Can you work these out from the model? Positions are in its coordinate system, mm. Give positions to 0.01 mm unless a question says otherwise; leave off trailing zeros. Write each loop counter-clockwise with the first axis right and the second up, starting at its lowest first coordinate (ties: lowest second). Pieces come first, ordered by that corner, then holes. Notation, with made-up numbers: (-34.75, 12.25) -> (-11.75, 12.25) arc R27 ccw to (-11.75, 33.25) -> close; hole circle Ø2 at (75, 10.5). An arc over 180 degrees is marked (long way). One line per item, written item: value.
from build123d import *

# Parameters (mm, degrees)
SKETCH3_R           = 19.3675
BOSS_EXTRUDE2_DEPTH = 50.8


with BuildPart() as part:
    # Sketch3 → Boss-Extrude2 (new body)
    with BuildSketch(Plane(origin=(0, 0, 0), x_dir=(1, 0, 0), z_dir=(0, 1, 0))):
        Circle(SKETCH3_R)
        with BuildLine():
            Line((1.905, 12.877355367), (1.905, 10.63625))
            Line((1.905, 10.63625), (-1.905, 10.63625))
            Line((-1.905, 10.63625), (-1.905, 12.877355367))
            ThreePointArc((-1.905, 12.877355367), (-4.981581581, 12.026601814), (-7.758626886, 10.452703722))
            Line((-7.758626886, 10.452703722), (-6.173926083, 8.86800292))
            Line((-6.173926083, 8.86800292), (-8.86800292, 6.173926083))
            Line((-8.86800292, 6.173926083), (-10.452703722, 7.758626886))
            ThreePointArc((-10.452703722, 7.758626886), (-12.026601814, 4.981581581), (-12.877355367, 1.905))
            Line((-12.877355367, 1.905), (-10.63625, 1.905))
            Line((-10.63625, 1.905), (-10.63625, -1.905))
            Line((-10.63625, -1.905), (-12.877355367, -1.905))
            ThreePointArc((-12.877355367, -1.905), (-12.026601814, -4.981581581), (-10.452703722, -7.758626886))
            Line((-10.452703722, -7.758626886), (-8.86800292, -6.173926083))
            Line((-8.86800292, -6.173926083), (-6.173926083, -8.86800292))
            Line((-6.173926083, -8.86800292), (-7.758626886, -10.452703722))
            ThreePointArc((-7.758626886, -10.452703722), (-4.981581581, -12.026601814), (-1.905, -12.877355367))
            Line((-1.905, -12.877355367), (-1.905, -10.63625))
            Line((-1.905, -10.63625), (1.905, -10.63625))
            Line((1.905, -10.63625), (1.905, -12.877355367))
            ThreePointArc((1.905, -12.877355367), (4.981581581, -12.026601814), (7.758626886, -10.452703722))
            Line((7.758626886, -10.452703722), (6.173926083, -8.86800292))
            Line((6.173926083, -8.86800292), (8.86800292, -6.173926083))
            Line((8.86800292, -6.173926083), (10.452703722, -7.758626886))
            ThreePointArc((10.452703722, -7.758626886), (12.026601814, -4.981581581), (12.877355367, -1.905))
            Line((12.877355367, -1.905), (10.63625, -1.905))
            Line((10.63625, -1.905), (10.63625, 1.905))
            Line((10.63625, 1.905), (12.877355367, 1.905))
            ThreePointArc((12.877355367, 1.905), (12.026601814, 4.981581581), (10.452703722, 7.758626886))
            Line((10.452703722, 7.758626886), (8.86800292, 6.173926083))
            Line((8.86800292, 6.173926083), (6.173926083, 8.86800292))
            Line((6.173926083, 8.86800292), (7.758626886, 10.452703722))
            ThreePointArc((7.758626886, 10.452703722), (4.981581581, 12.026601814), (1.905, 12.877355367))
        make_face(mode=Mode.SUBTRACT)
    extrude(amount=BOSS_EXTRUDE2_DEPTH)


solid = part.part
1) Will these pins go through, and if not, where does the flat tip stop? pin 1 (1.5 mm diameter, centred on y = 41.5, z = 11, fed in from +X); pin 2 (1.1 mm diameter, centred on y = 19, z = -11.5, fed in from +X); pin 3 (5 mm diameter, centred on y = 14, z = 11, fed in from -X); pin 4 (2 mm diameter, centred on x = 11.5, z = 8, fed in from -Y).
Answer list:
pin 1: stops at x = 16.43
pin 2: stops at x = 15.97
pin 3: stops at x = -17.4
pin 4: stops at y = 0
2) If we section it at D-D (x = 16.5): Write out the boundary of the cut face in (y, z).
Answer list:
outline: (0, -10.14) -> (50.8, -10.14) -> (50.8, 10.14) -> (0, 10.14) -> close
3) If we section it at B-B (x = 0): Write out the boundary of the cut face in (y, z).
Answer list:
outline: (0, -19.37) -> (50.8, -19.37) -> (50.8, -10.64) -> (0, -10.64) -> close; (0, 10.64) -> (50.8, 10.64) -> (50.8, 19.37) -> (0, 19.37) -> close
4) If we section it at A-A (z = 0): Write out the boundary of the cut face in (x, y), and give its area (3 significant figures).
Answer list:
outline: (-19.37, 0) -> (-10.64, 0) -> (-10.64, 50.8) -> (-19.37, 50.8) -> close; (10.64, 0) -> (19.37, 0) -> (19.37, 50.8) -> (10.64, 50.8) -> close
area: 887 mm^2
5) I need wall thicknesses on L1, parallel to X at y = 38.5, z = -0.5; L2, parallel to X at y = 43, z = 7. Which ranges of each line are inside material? Lowest first, please.
Answer list:
L1: x = -19.36 to -10.64, 10.64 to 19.36
L2: x = -18.06 to -10.98, -9.69 to -8.04, 8.04 to 9.69, 10.98 to 18.06
